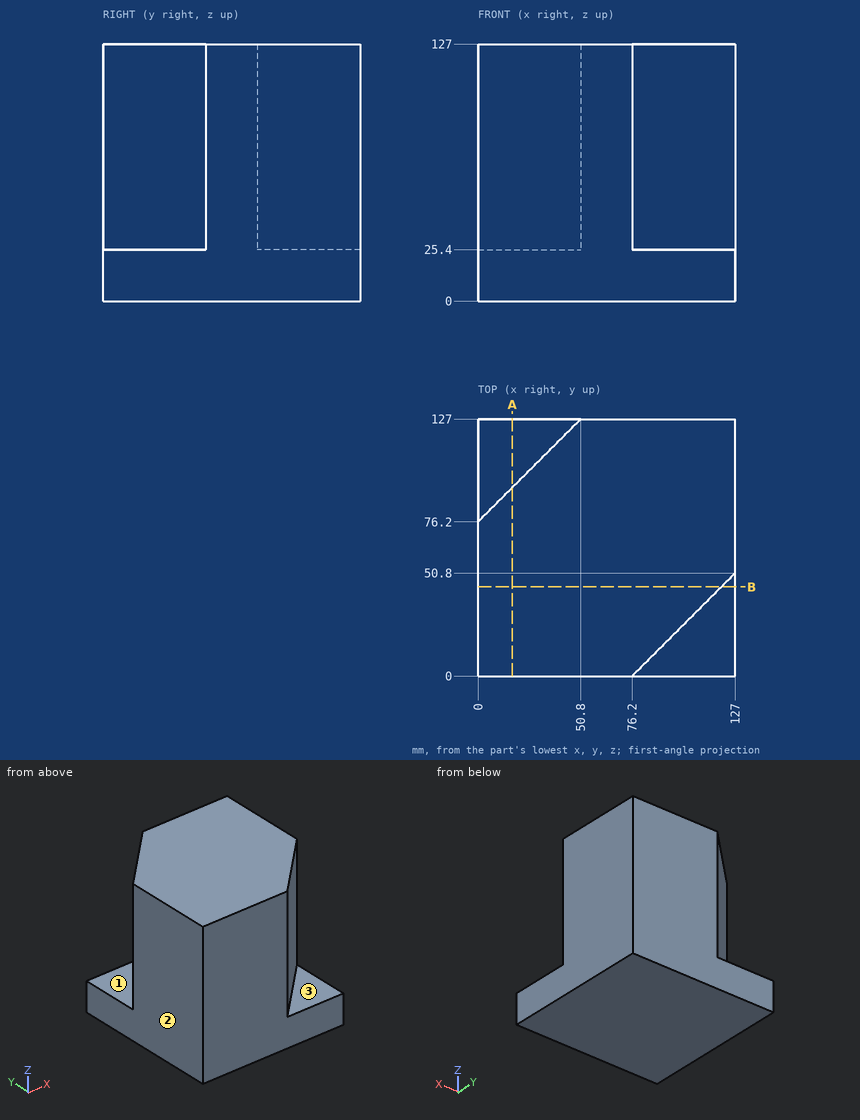
Could you check a few things on this drawing? It's one solid part, dimensions in mm from its lowest x, y, z. A direction names the side the tool comes from. Coordinates: 2 decimals unless noted, no trailing zeros. Write each loop counter-clockwise with the first axis right and the second up, starting at its lowest first coordinate (ties: lowest second). Pieces come first, ordered by that corner, then holes. Notation, with made-up numbers: (-12, 62.5) - (4, 62.5) arc R10 ccw to (4, 69.5) - close; hole circle Ø11 at (-25.75, 35). An arc over 180 degrees is marked (long way). Put each result on its own line as item: value. Start each with the question number.
Q1. I want a section at A-A on x = 17. Write out the boundary of the cut face in (y, z).
Q2. I want a section at B-B on y = 44. Write out the boundary of the cut face in (x, z), plus the area to 3 significant figures.
Q3. I'm going to push flat-ended pins straight in: P1, Ø8, axis at y = 82.5, z = 107, coming from the -X side; P2, Ø5, axis at x = 25.5, z = 57.5, coming from the +Y side; P3, Ø4, axis at y = 48, z = 31, coming from the +X side. Where does each tip first touch, or does it pass through?
Q4. Please list where these lines run through material, in increasing order: L1, parallel to Y at x = 116, z = 36.5; L2, parallel to Y at x = 43, z = 52.5; L3, parallel to X at y = 16.5, z = 91.
Q5. Which directions (+Z, -Z, +X, -X, +Y, -Y) give clear straight access to the entire face, cutting with the end or side of a thin tool? Please do the marked faces 1, 2 and 3.
Checks:
1. outline: (0, 0) - (127, 0) - (127, 25.4) - (93.2, 25.4) - (93.2, 127) - (0, 127) - close
2. outline: (0, 0) - (127, 0) - (127, 25.4) - (120.2, 25.4) - (120.2, 127) - (0, 127) - close
2. area: 15,400 mm²
3. P1: x = 2.3
3. P2: y = 104.2
3. P3: x = 126.2
4. L1: 39.8 to 127
4. L2: 0 to 119.2
4. L3: 0 to 92.7
5. face 1: +Z, -X, +Y
5. face 2: +Z, -Z, -X, +Y, -Y
5. face 3: +Z, +X, -Y
